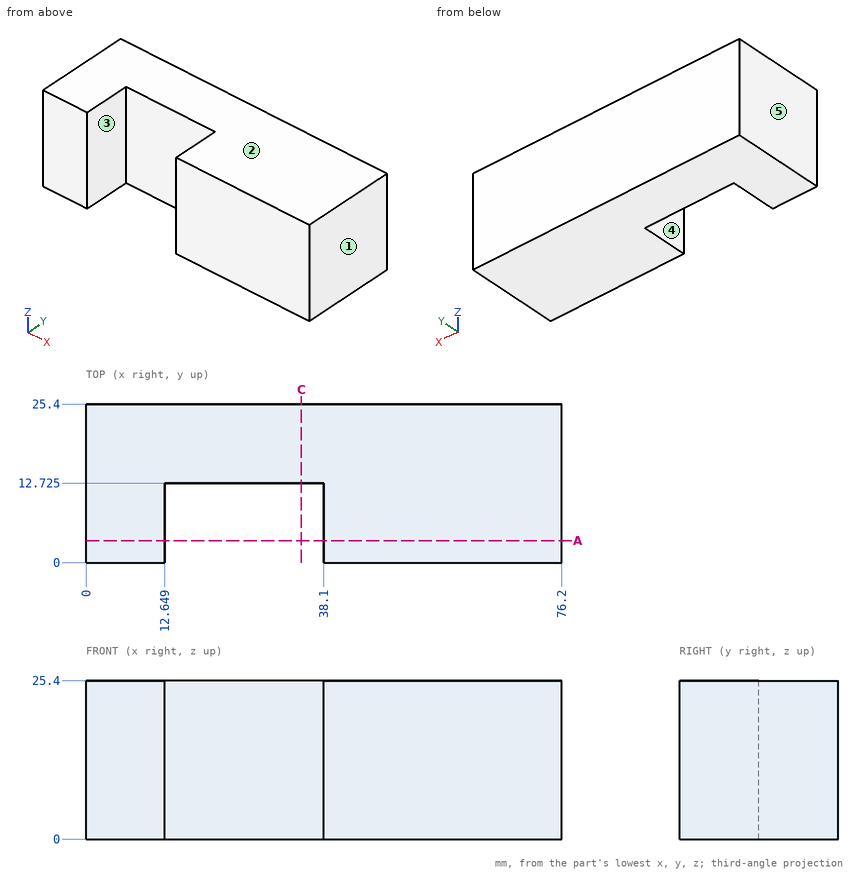
Design review of the part shown in the three views and the two pictorial views. Dimensions are in mm from the part's minimum x, y and z. A direction names the side the tool comes from. Round coordinates to 2 decimals unless told otherwise and drop trailing zeros. Write each loop counter-clockwise with the first axis right and the second up, starting at its lowest first coordinate (ties: lowest second). Pieces come first, ordered by that corner, then holes. Notation, with made-up numbers: M 69,-6 L 95,-6 A19 cw 95,23 Z; hole C -3.75,-11 d7. An arc over 180 degrees is marked long. One line per item, written item: value. Start each with the question number.
1. Take a section at C-C on x = 34.5. State the section outline as (y, z) points (1 decimal).
2. To check wall thickness, follow probe 1 along X at (y, z) = (2, 14); probe 2 along Y at (x, z) = (35.5, 16) (1 decimal). State the ranges of each line that lie inside material, in increasing order. Write a range as from..to.
3. Clearance check with a flat-ended pin moving along its axis: P1, Ø3, axis at x = 21.5, z = 8.5, coming from the -Y side (1 decimal). State where the tip first meets the part, or that it passes through.
4. Take a section at A-A on y = 3.5. State the section outline as (x, z) points.
5. Draft analysis for pull direction X (two halves, no side actions). For the marked faces 1, 2 and 3, state which applies: pulls with the +X half, pulls with the -X half, needs draft (parallel to the pull), parting line crosses it, or undercut.
6. For the marked faces 4 and 5, list the 3-axis set-ups (+Z, -Z, +X, -X, +Y, -Y) from which the entire face can be reached by the end or side of a thin tool; tool diameter is ignored.
Computed:
1. outline: M 12.7,0 L 25.4,0 L 25.4,25.4 L 12.7,25.4 Z
2. probe 1: x = 0..12.65, 38.1..76.2
2. probe 2: y = 12.7..25.4
3. P1: stops at y = 12.7
4. outline: M 0,0 L 12.65,0 L 12.65,25.4 L 0,25.4 Z; M 38.1,0 L 76.2,0 L 76.2,25.4 L 38.1,25.4 Z
5. face 1: pulls with the +X half
5. face 2: needs draft
5. face 3: undercut
6. face 4: +Z, -Z, -Y
6. face 5: +Z, -Z, -X, +Y, -Y
